```python
from build123d import *

# Parameters (mm, degrees)
SKETCH1_W           = 300
SKETCH1_H           = 150
SKETCH1_R           = 14.235
BOSS_EXTRUDE1_DEPTH = 3
CUT_EXTRUDE1_REACH  = 5
SKETCH2_R           = 3.225
SKETCH4_R           = 2.0193
CUT_EXTRUDE4_DEPTH  = 4
CUT_EXTRUDE5_DEPTH  = 4
CUT_EXTRUDE6_DEPTH  = 10
SKETCH7_R           = 2.75
CUT_EXTRUDE7_DEPTH  = 4


with BuildPart() as part:
    # Sketch1 → Boss-Extrude1 (new body)
    with BuildSketch(Plane(origin=(0, 0, 0), x_dir=(0, 0, -1), z_dir=(1, 0, 0))):
        with Locations((150, 75)):
            Rectangle(SKETCH1_W, SKETCH1_H)
        with Locations((30, 55)):
            Circle(SKETCH1_R, mode=Mode.SUBTRACT)
    extrude(amount=BOSS_EXTRUDE1_DEPTH)

    # Sketch2 → Cut-Extrude1 (cut, up to next)
    with BuildSketch(Plane.ZY, mode=Mode.PRIVATE) as cut_extrude1_sk1:
        with Locations((-10, 110)):
            Circle(SKETCH2_R)
    cut_extrude1_tool1 = extrude(cut_extrude1_sk1.sketch, amount=-CUT_EXTRUDE1_REACH, mode=Mode.PRIVATE) & part.part
    add(cut_extrude1_tool1.solids().sort_by_distance((0, 110, -10))[0], mode=Mode.SUBTRACT)
    # Sketch2 → Cut-Extrude1 (cut, up to next)
    with BuildSketch(Plane.ZY, mode=Mode.PRIVATE) as cut_extrude1_sk2:
        with BuildLine():
            Line((-236, 104.938413591), (-216, 104.938413591))
            ThreePointArc((-216, 104.938413591), (-212.77, 101.708413591), (-216, 98.478413591))
            Line((-216, 98.478413591), (-236, 98.478413591))
            ThreePointArc((-236, 98.478413591), (-239.23, 101.708413591), (-236, 104.938413591))
        make_face()
    cut_extrude1_tool2 = extrude(cut_extrude1_sk2.sketch, amount=-CUT_EXTRUDE1_REACH, mode=Mode.PRIVATE) & part.part
    add(cut_extrude1_tool2.solids().sort_by_distance((0, 101.708414, -226))[0], mode=Mode.SUBTRACT)
    # Sketch2 → Cut-Extrude1 (cut, up to next)
    with BuildSketch(Plane.ZY, mode=Mode.PRIVATE) as cut_extrude1_sk3:
        with BuildLine():
            Line((-216, 16.231694356), (-236, 16.231694356))
            ThreePointArc((-236, 16.231694356), (-239.225, 19.456694356), (-236, 22.681694356))
            Line((-236, 22.681694356), (-216, 22.681694356))
            ThreePointArc((-216, 22.681694356), (-212.775, 19.456694356), (-216, 16.231694356))
        make_face()
    cut_extrude1_tool3 = extrude(cut_extrude1_sk3.sketch, amount=-CUT_EXTRUDE1_REACH, mode=Mode.PRIVATE) & part.part
    add(cut_extrude1_tool3.solids().sort_by_distance((0, 19.456694, -226))[0], mode=Mode.SUBTRACT)

    # Sketch4 → Cut-Extrude4 (cut, through all)
    with BuildSketch(Plane(origin=(3, 0, 0), x_dir=(0, 0, -1), z_dir=(1, 0, 0))):
        with Locations((12.039487758, 37.039487758)):
            Circle(SKETCH4_R)
        with Locations((12.039487758, 72.960512242)):
            Circle(SKETCH4_R)
        with Locations((4.6, 55)):
            Circle(SKETCH4_R)
        with Locations((47.960512242, 37.039487758)):
            Circle(SKETCH4_R)
        with Locations((55.4, 55)):
            Circle(SKETCH4_R)
        with Locations((47.960512242, 72.960512242)):
            Circle(SKETCH4_R)
    extrude(amount=-CUT_EXTRUDE4_DEPTH, mode=Mode.SUBTRACT)

    # Sketch5 → Cut-Extrude5 (cut, through all)
    with BuildSketch(Plane.ZY):
        Polygon((-71, 0), (-71, 9), (0, 35), (0, 0), align=None)
        Polygon((0, 85.848631797), (-186.802640374, 119.641480316), (-300.310491503, 119.641480316), (-300.310491503, 150), (0, 150), align=None)
    extrude(amount=-CUT_EXTRUDE5_DEPTH, mode=Mode.SUBTRACT)

    # Sketch6 → Cut-Extrude6 (cut)
    with BuildSketch(Plane.ZY):
        Polygon((-250.717958721, 165.712896148), (-250.717958721, 16.875947155), (-228.92403237, 9), (-228.92403237, 0), (-355.768886916, 0), (-364.830865455, 165.712896148), align=None)
    extrude(amount=-CUT_EXTRUDE6_DEPTH, mode=Mode.SUBTRACT)

    # Sketch7 → Cut-Extrude7 (cut, through all)
    with BuildSketch(Plane(origin=(3, 0, 0), x_dir=(0, 0, -1), z_dir=(1, 0, 0))):
        with Locations((89.962016185, 5)):
            Circle(SKETCH7_R)
        with Locations((149.962016185, 5)):
            Circle(SKETCH7_R)
        with Locations((209.962016185, 5)):
            Circle(SKETCH7_R)
    extrude(amount=-CUT_EXTRUDE7_DEPTH, mode=Mode.SUBTRACT)


solid = part.part
```
Check sheet for the modelled part. Datum: model origin and axes. Units: mm. Round coordinates to 2 decimals unless told otherwise and drop trailing zeros. Loops run counter-clockwise (first coordinate to the right, second up) from the corner with the lowest first, then second, coordinate; pieces in that order, holes last. Notation, with made-up numbers: (-23, 18.25) -> (-14, 18.25) arc R21 cw to (-14, 45.25) -> close; hole circle Ø6 at (80, 14.25). An arc over 180 degrees is marked (long way). Write item = value, one per line. Start each with the question number.
1) Release check for a two-part mould opening along Z. For faces 1 (the flat face through (1.48, 12.99, -239.97)), 2 (the cylindrical face through (1.521, 3.947, -152.502)), 3 (the flat face through (3, 61, -124)) record: released by +Z, released by -Z, zero draft, split by the parting line, or undercut.
2) Gauge pin test, flat ends, axial feed: pin 1 Ø0.9 at (x, y) = (1.5, 2.5) entering from +Z; pin 2 Ø0.9 at (x, y) = (1.5, 6.5) entering from -Z. Record the tip position at first contact, or that the pin passes through.
3) Sectioned sample at C-C, the plane x = 2.35. State how many separate pieces and enclosed holes the cut face has, plus the area to 3 significant figures.
4) Sectioned sample at D-D, the plane z = -96.5. Record the cut outline in (x, y).
5) Sectioned sample at A-A, the plane y = 5. Record the cut outline in (x, z), plus the area to 3 significant figures.
6) Thickness scan on probe 1 along Y at (x, z) = (1.95, -228.5); probe 2 along Y at (x, z) = (2.55, -47); probe 3 along Z at (x, y) = (2.15, 61). Record the ranges inside material, lowest first.
7) Sectioned sample at B-B, the plane z = -30. Record the cut outline in (x, y) (3 decimals).
Results are:
q1.face_1 = released by -Z
q1.face_2 = undercut
q1.face_3 = zero draft
q2.pin_1 = -71
q2.pin_2 = -228.92
q3.separate_pieces = 1
q3.enclosed_holes = 12
q3.area = 23,900 mm^2
q4.outline = (0, 0) -> (3, 0) -> (3, 103.31) -> (0, 103.31) -> close
q5.outline = (0, -228.92) -> (3, -228.92) -> (3, -212.71) -> (0, -212.71) -> close; (0, -207.21) -> (3, -207.21) -> (3, -152.71) -> (0, -152.71) -> close; (0, -147.21) -> (3, -147.21) -> (3, -92.71) -> (0, -92.71) -> close; (0, -87.21) -> (3, -87.21) -> (3, -71) -> (0, -71) -> close
q5.area = 424 mm^2
q6.probe_1 = 0 to 16.23, 22.68 to 98.48, 104.94 to 119.64
q6.probe_2 = 17.79 to 35.26, 38.82 to 71.18, 74.74 to 94.35
q6.probe_3 = -250.72 to -42.91, -17.09 to 0
q7.outline = (0, 24.014) -> (3, 24.014) -> (3, 40.765) -> (0, 40.765) -> close; (0, 69.235) -> (3, 69.235) -> (3, 91.276) -> (0, 91.276) -> close
